```python
from build123d import *

# Parameters (mm, degrees)
BOSS_EXTRUDE1_DEPTH = 6.35
SKETCH2_R           = 2.921
CUT_EXTRUDE1_DEPTH  = 210.55
SKETCH3_W           = 5.08
SKETCH3_H           = 50.8
CUT_EXTRUDE2_DEPTH  = 210.55
FILLET1_R           = 12.7
SKETCH4_W           = 3.175
SKETCH4_H           = 15.875
CUT_EXTRUDE3_DEPTH  = 205.627703159
FILLET2_R           = 1.524


with BuildPart() as part:
    # Sketch1 → Boss-Extrude1 (new body)
    with BuildSketch(Plane.XY):
        Polygon((0, 0), (0, 50.8), (25.4, 50.8), (25.4, 25.4), (177.8, 25.4), (177.8, 50.8), (203.2, 50.8), (203.2, 0), align=None)
    extrude(amount=BOSS_EXTRUDE1_DEPTH)

    # Sketch2 → Cut-Extrude1 (cut, through all)
    with BuildSketch(Plane.XY.offset(6.35)):
        with Locations((12.7, 38.1)):
            Circle(SKETCH2_R)
        with Locations((12.7, 12.7)):
            Circle(SKETCH2_R)
        with Locations((38.1, 12.7)):
            Circle(SKETCH2_R)
        with Locations((63.5, 12.7)):
            Circle(SKETCH2_R)
        with Locations((88.9, 12.7)):
            Circle(SKETCH2_R)
        with Locations((114.3, 12.7)):
            Circle(SKETCH2_R)
        with Locations((139.7, 12.7)):
            Circle(SKETCH2_R)
        with Locations((165.1, 12.7)):
            Circle(SKETCH2_R)
        with Locations((190.5, 12.7)):
            Circle(SKETCH2_R)
        with Locations(Location((190.5, 38.1, 0), (0, 0, 180))):
            Circle(SKETCH2_R)
    extrude(amount=-CUT_EXTRUDE1_DEPTH, mode=Mode.SUBTRACT)

    # Sketch3 → Cut-Extrude2 (cut, through all)
    with BuildSketch(Plane.XY.offset(6.35)):
        with Locations((2.54, 25.4)):
            Rectangle(SKETCH3_W, SKETCH3_H)
        with Locations((200.66, 25.4)):
            Rectangle(SKETCH3_W, SKETCH3_H)
    extrude(amount=-CUT_EXTRUDE2_DEPTH, mode=Mode.SUBTRACT)

    # Fillet1
    fillet1_edges = [part.edges().sort_by_distance(p)[0] for p in [
        (25.4, 25.4, 3.175),
        (177.8, 25.4, 3.175),
    ]]
    fillet(fillet1_edges, radius=FILLET1_R)

    # Sketch4 → Cut-Extrude3 (cut, through all)
    with BuildSketch(Plane.XY.offset(6.35)):
        with Locations((6.6675, 19.05)):
            Rectangle(SKETCH4_W, SKETCH4_H)
        with Locations((196.5325, 19.05)):
            Rectangle(SKETCH4_W, SKETCH4_H)
    extrude(amount=-CUT_EXTRUDE3_DEPTH, mode=Mode.SUBTRACT)

    # Fillet2
    fillet2_edges = [part.edges().sort_by_distance(p)[0] for p in [
        (5.08, 11.1125, 3.175),
        (5.08, 26.9875, 3.175),
        (8.255, 26.9875, 3.175),
        (8.255, 11.1125, 3.175),
        (198.12, 11.1125, 3.175),
        (194.945, 11.1125, 3.175),
        (194.945, 26.9875, 3.175),
        (198.12, 26.9875, 3.175),
    ]]
    fillet(fillet2_edges, radius=FILLET2_R)


solid = part.part
```
Geometry: final body of the model. Coordinates: model frame, mm. A direction names the side the tool comes from. Round coordinates to 2 decimals unless told otherwise and drop trailing zeros. Write each loop counter-clockwise with the first axis right and the second up, starting at its lowest first coordinate (ties: lowest second). Pieces come first, ordered by that corner, then holes. Notation, with made-up numbers: (30, 55) -> (73, 55) arc R8 cw to (73, 59) -> close; hole circle Ø2 at (-12.75, 10). An arc over 180 degrees is marked (long way). Use CSV: the item, a comma, the result in double quotes. Start each with the question number.
Q1. Section D-D (z = 2.5). Give the number of separate pieces and of enclosed holes in the cut face, plus the area to 3 significant figures.
Q2. Pull-direction query (X, two-part tool) for faces 1 (the face through (103, 0, 3)), 2 (the face through (198.12, 39, 3)), 3 (the face through (14.05, 35.51, 3.22)); classes: pulls with the +X half, pulls with the -X half, needs draft (parallel to the pull), parting line crosses it, or undercut.
Q3. Section A-A (y = 45). Return loops of the section in (x, z), plus the area to 3 significant figures.
Q4. Section B-B (x = 190.5). Return loops of the section in (y, z).
Q5. Line query: L1, parallel to Y at x = 12.7, z = 3.25; L2, parallel to X at y = 48.5, z = 2.5; L3, parallel to Y at x = 53, z = 3. Output: solid intervals per line, ascending.
Q6. First-contact query: pin 1 Ø3 at (x, z) = (99.5, 4.5) entering from +Y; pin 2 Ø5.5 at (x, y) = (190.5, 12.7) entering from +Z; pin 3 Ø1.9 at (y, z) = (22, 4.5) entering from -X (3 decimals). Flat tips, straight axial feed; report the tip coordinate or a pass-through.
Q7. Section C-C (x = 139.7). Return loops of the section in (y, z), plus the area to 3 significant figures.
Q8. Reachability of faces 4 (the face through (5.08, 5, 3)), 5 (the face through (162.18, 12.83, 3.22)), 6 (the face through (177.8, 44, 3)), 7 (the face through (194.945, 19, 3)), 8 (the face through (8.255, 19, 3)) from +Z, -Z, +X, -X, +Y, -Y: full face, straight path, thin tool, end or side. Return the list, or none.
Result sheet:
1,separate pieces,"1"
1,enclosed holes,"10"
1,area,"5,640 mm²"
2,face 1,"needs draft"
2,face 2,"pulls with the +X half"
2,face 3,"undercut"
3,outline,"(5.08, 0) -> (25.4, 0) -> (25.4, 6.35) -> (5.08, 6.35) -> close; (177.8, 0) -> (198.12, 0) -> (198.12, 6.35) -> (177.8, 6.35) -> close"
3,area,"258 mm²"
4,outline,"(0, 0) -> (9.78, 0) -> (9.78, 6.35) -> (0, 6.35) -> close; (15.62, 0) -> (35.18, 0) -> (35.18, 6.35) -> (15.62, 6.35) -> close; (41.02, 0) -> (50.8, 0) -> (50.8, 6.35) -> (41.02, 6.35) -> close"
5,L1,"0 to 9.78, 15.62 to 35.18, 41.02 to 50.8"
5,L2,"5.08 to 25.4, 177.8 to 198.12"
5,L3,"0 to 25.4"
6,pin 1,"y = 25.4"
6,pin 2,"through"
6,pin 3,"x = 8.255"
7,outline,"(0, 0) -> (9.78, 0) -> (9.78, 6.35) -> (0, 6.35) -> close; (15.62, 0) -> (25.4, 0) -> (25.4, 6.35) -> (15.62, 6.35) -> close"
7,area,"124 mm²"
8,face 4,"+Z, -Z, -X, +Y, -Y"
8,face 5,"+Z, -Z"
8,face 6,"+Z, -Z, +Y"
8,face 7,"+Z, -Z, +X"
8,face 8,"+Z, -Z, -X"
